Geometry: final body of the model. Coordinates: model frame, mm. A direction names the side the tool comes from. Give positions to 0.01 mm unless a question says otherwise; leave off trailing zeros. Loops run counter-clockwise (first coordinate to the right, second up) from the corner with the lowest first, then second, coordinate; pieces in that order, holes last. Notation, with made-up numbers: (12.5, 45) -> (25.5, 45) arc R22 cw to (25.5, 60) -> close; hole circle Ø4 at (46, -33.5). An arc over 180 degrees is marked (long way). One line per question, with ' | ' between items. Start each with the question number.
Item 1: Section A-A on x = 0. Return loops of the section in (y, z), then the cut area to 3 significant figures.
Item 2: Set-up query: faces 4 (the cylindrical face through (9.139, 14.334, -2.465)), 5 (the cylindrical face through (-18.61, 18.51, 2.54)). Return all of +Z, -Z, +X, -X, +Y, -Y with unobstructed straight access to the full face (end or side cutting, diameter ignored); none if empty.
Item 3: Section C-C on z = 1.25. Return loops of the section in (x, y).
Item 4: Pin query (flat end, axial travel): P1, Ø3.5, axis at x = 17.5, y = -17.5, coming from the -Z side; P2, Ø1, axis at x = -8, z = -1, coming from the +Y side. Return the tip coordinate at first contact, or that it passes through.
Item 5: Section D-D on y = 15. Return loops of the section in (x, z).
Item 6: Material intervals for line 1 along Y through (x, z) = (-17.5, 2.55); line 2 along Y through (x, z) = (17, 1.75), sorted ascending. Write a range as [from, to].
Item 7: Mould query, pull axis Y, two halves, no side actions, for faces 1 (the cylindrical face through (16, 17.57, 2.54)), 2 (the flat face through (25, 0, 2)), 3 (the flat face through (0, -25, 2)). Classes: released by +Y, released by -Y, zero draft, split by the parting line, or undercut.
from build123d import *

# Parameters (mm, degrees)
SKETCH1_R           = 17
SKETCH1_R_2         = 12
BOSS_EXTRUDE1_DEPTH = 5
SKETCH2_W           = 50
SKETCH2_H           = 50
BOSS_EXTRUDE2_DEPTH = 5
SKETCH3_R           = 5
CUT_EXTRUDE1_DEPTH  = 37.742346142
SKETCH4_R           = 1.5
CUT_EXTRUDE2_DEPTH  = 37.742346142


with BuildPart() as part:
    # Sketch1 → Boss-Extrude1 (new body)
    with BuildSketch(Plane.XY):
        Circle(SKETCH1_R)
        Circle(SKETCH1_R_2, mode=Mode.SUBTRACT)
    extrude(amount=-BOSS_EXTRUDE1_DEPTH)

    # Sketch2 → Boss-Extrude2 (add)
    with BuildSketch(Plane.XY):
        Rectangle(SKETCH2_W, SKETCH2_H)
    extrude(amount=BOSS_EXTRUDE2_DEPTH)

    # Sketch3 → Cut-Extrude1 (cut, through all)
    with BuildSketch(Plane.XY.offset(5)):
        Circle(SKETCH3_R)
    extrude(amount=-CUT_EXTRUDE1_DEPTH, mode=Mode.SUBTRACT)

    # Sketch4 → Cut-Extrude2 (cut, through all)
    with BuildSketch(Plane.XY.offset(5)):
        with Locations((-17.5, 17.5)):
            Circle(SKETCH4_R)
        with Locations((17.5, 17.5)):
            Circle(SKETCH4_R)
        with Locations((-17.5, -17.5)):
            Circle(SKETCH4_R)
        with Locations((17.5, -17.5)):
            Circle(SKETCH4_R)
    extrude(amount=-CUT_EXTRUDE2_DEPTH, mode=Mode.SUBTRACT)


solid = part.part
Result sheet:
1) outline: (-25, 0) -> (-17, 0) -> (-17, -5) -> (-12, -5) -> (-12, 0) -> (-5, 0) -> (-5, 5) -> (-25, 5) -> close; (5, 0) -> (12, 0) -> (12, -5) -> (17, -5) -> (17, 0) -> (25, 0) -> (25, 5) -> (5, 5) -> close | area: 250 mm²
2) face 4: -Z | face 5: +Z, -Z
3) outline: (-25, -25) -> (25, -25) -> (25, 25) -> (-25, 25) -> close; hole circle Ø3 at (-17.5, -17.5); hole circle Ø3 at (-17.5, 17.5); hole circle Ø10 at (0, 0); hole circle Ø3 at (17.5, -17.5); hole circle Ø3 at (17.5, 17.5)
4) P1: stops at z = 0 | P2: stops at y = 15.26
5) outline: (-25, 0) -> (-8, 0) -> (-8, -5) -> (8, -5) -> (8, 0) -> (25, 0) -> (25, 5) -> (-25, 5) -> close
6) line 1: y = [-25, -19], [-16, 16], [19, 25] | line 2: y = [-25, -18.91], [-16.09, 16.09], [18.91, 25]
7) face 1: undercut | face 2: zero draft | face 3: released by -Y
